Autodesk Inventor part; units mm, degrees
ref_plane "YZ Plane" through (0, 0, 0) normal (1, 0, 0) x (0, 1, 0)
ref_plane "XZ Plane" through (0, 0, 0) normal (0, 1, 0) x (-1, 0, 0)
ref_plane "XY Plane" through (0, 0, 0) normal (0, 0, 1) x (1, 0, 0)
sketch "Sketch1" plane through (0, 0, 0) normal (0, 0, 1) x (1, 0, 0)
  line L0 (-40, 60) -> (40, 60)
  line L1 (40, 60) -> (40, -60)
  line L2 (40, -60) -> (-40, -60)
  line L3 (-40, -60) -> (-40, 60)
  line L4 (-40, 60) -> (40, -60) construction
  line L5 (40, 60) -> (-40, -60) construction
  point P0 (0, 0)
  dimension "d0" = 80
  dimension "d1" = 120
extrude "Extrusion1" add sketch "Sketch1" along normal blind 3
sketch "Sketch2" plane through (0, 0, 3) normal (0, 0, 1) x (1, 0, 0)
  line L0 (-40, -60) -> (40, -60)
  line L1 (-40, 60) -> (-40, -60)
  point P0 (0, 0)
  point P1 (-30, -39)
  point P2 (30, -39)
  point P3 (-30, 1)
  point P4 (30, 1)
  dimension "d4" = 21
  dimension "d5" = 10
  dimension "d6" = 40
  dimension "d7" = 60
hole "Hole1" at (-30, -39, 3) at (30, -39, 3) at (-30, 1, 3) at (30, 1, 3) direction (0, 0, -1) diameter 5.1 end through all
sketch "Sketch3" plane through (0, 0, 3) normal (0, 0, 1) x (1, 0, 0)
  circle A0 centre (0, 38) radius 11
  point P0 (0, 0)
  dimension "d15" = 22
  dimension "d16" = 38
extrude "Extrusion2" cut sketch "Sketch3" against normal through all
sketch "Sketch4" plane through (0, 0, 3) normal (0, 0, 1) x (1, 0, 0)
  circle A0 centre (0, 38) radius 11
  line L0 (-15.5, 53.5) -> (15.5, 53.5)
  line L1 (15.5, 53.5) -> (15.5, 22.5)
  line L2 (15.5, 22.5) -> (-15.5, 22.5)
  line L3 (-15.5, 22.5) -> (-15.5, 53.5)
  line L4 (-15.5, 53.5) -> (15.5, 22.5) construction
  line L5 (15.5, 53.5) -> (-15.5, 22.5) construction
  point P0 (0, 0)
  dimension "d19" = 31
  dimension "d20" = 31
hole "Hole2" at (-15.5, 53.5, 3) at (-15.5, 22.5, 3) at (15.5, 22.5, 3) at (15.5, 53.5, 3) direction (0, 0, -1) diameter 3.5 end through all
sketch "Sketch5" plane through (0, 0, 3) normal (0, 0, 1) x (1, 0, 0)
  line L0 (40, 60) -> (-40, 60)
  line L1 (-22, 60) -> (-40, 15)
  line L2 (-40, 60) -> (-40, -60)
  line L3 (22, 60) -> (40, 15)
  line L4 (40, -60) -> (40, 60)
  point P0 (0, 0)
  dimension "d28" = 15
  dimension "d29" = 15
  dimension "d30" = 18
  dimension "d31" = 18
  dimension "d32" = 44
extrude "Extrusion3" cut sketch "Sketch5" against normal through all
sketch "Sketch7" plane through (0, 0, 0) normal (0, 0, -1) x (-1, 0, 0)
  line L0 (40, -60) -> (-40, -60)
  point P0 (0, 0)
  point P1 (0, -39.5)
  dimension "d41" = 20.5
hole "Hole3" at (0, -39.5, 0) direction (0, 0, 1) diameter 4.5 end through all
chamfer "Chamfer1" distance 12 angle 45 2 edges at (-40, -60, 1.5) (40, -60, 1.5)
sketch "Sketch11" plane through (0, 0, 3) normal (0, 0, 1) x (1, 0, 0)
  line L0 (-28, -60) -> (28, -60)
  circle A0 centre (0, 38) radius 11
  point P0 (0, 0)
  point P1 (0, 8)
  point P2 (0, -53)
  dimension "d67" = 7
  dimension "d68" = 30
hole "Hole5" at (0, 8, 3) at (0, -53, 3) direction (0, 0, -1) diameter 4.5 end through all
equation "\"d31\" = d30"
properties part number "Z-Axis - Back Plate"
Design review of the part built by this model. Coordinates are the model's own, in mm. Coordinates: 2 decimals unless noted, no trailing zeros. Write each loop counter-clockwise with the first axis right and the second up, starting at its lowest first coordinate (ties: lowest second). Pieces come first, ordered by that corner, then holes.
1) Insertion check: pin 1 (6 mm diameter, centred on x = 0, y = 8, fed in from -Z); pin 2 (4 mm diameter, centred on x = 30, y = -39, fed in from +Z). Each pin has a flat end and moves straight along its axis. Give the tip position at first contact, or say it passes through.
2) Add section B-B (y = 8). Write out the cut boundary in (x, z), plus the area to 4 significant figures.
3) Add section D-D (z = 2.15). State how many separate pieces and enclosed holes the cut face has, plus the area to 3 significant figures.
4) Add section C-C (x = 15.5). Write out the cut boundary in (y, z), plus the area to 3 significant figures.
5) Add section A-A (x = 0). Write out the cut boundary in (y, z).
6) Mouldability with a two-part tool opening along Y and no side actions: class faces 1 (the flat face through (-1, 1, 3)), 2 (the cylindrical face through (-0.099, 10.248, 1.479)), 3 (the flat face through (0, 60, 1)) as +Y half, -Y half, draft (parallel to the pull), parting line (faces both ways), or undercut.
7) To check wall thickness, follow L1, parallel to X at y = 1, z = 0.9; L2, parallel to X at y = 22.5, z = 1.85; L3, parallel to Y at x = -17, z = 0.9. State the ranges of each line that lie inside material, in increasing order.
Check result:
1. pin 1: stops at z = 0
1. pin 2: passes through
2. outline: (-40, 0) - (-2.25, 0) - (-2.25, 3) - (-40, 3) - close; (2.25, 0) - (40, 0) - (40, 3) - (2.25, 3) - close
2. area: 226.5 mm2
3. separate pieces: 1
3. enclosed holes: 12
3. area: 8,100 mm2
4. outline: (-60, 0) - (20.75, 0) - (20.75, 3) - (-60, 3) - close; (24.25, 0) - (51.75, 0) - (51.75, 3) - (24.25, 3) - close; (55.25, 0) - (60, 0) - (60, 3) - (55.25, 3) - close
4. area: 339 mm2
5. outline: (-60, 0) - (-55.25, 0) - (-55.25, 3) - (-60, 3) - close; (-50.75, 0) - (-41.75, 0) - (-41.75, 3) - (-50.75, 3) - close; (-37.25, 0) - (5.75, 0) - (5.75, 3) - (-37.25, 3) - close; (10.25, 0) - (27, 0) - (27, 3) - (10.25, 3) - close; (49, 0) - (60, 0) - (60, 3) - (49, 3) - close
6. face 1: draft
6. face 2: undercut
6. face 3: +Y half
7. L1: x = -40 to -32.55, -27.45 to 27.45, 32.55 to 40
7. L2: x = -37 to -17.25, -13.75 to 13.75, 17.25 to 37
7. L3: y = -60 to 21.6, 23.4 to 52.6, 54.4 to 60
